Answer from the drawing. Dimensions are ordinates in mm from the lowest x, y and z of the part. Coordinates: 2 decimals unless noted, no trailing zeros. Write each loop counter-clockwise with the first axis right and the second up, starting at its lowest first coordinate (ties: lowest second). Pieces come first, ordered by that corner, then holes.
(1) The part is cut by section A-A on y = 1.8. Give the number of separate pieces and of enclosed holes in the cut face, plus the area to 3 significant figures.
(2) Straight lines are drawn through the part: line 1 (X direction, y = 0.6, z = 74.5) (1 decimal); line 2 (Z direction, x = 269, y = 0.55) (1 decimal). For each, find the intervals that lie inside material, in ascending order.
(3) Given P1, Ø1.6, axis at x = 264.5, y = 2, coming from the -Z side (3 decimals); P2, Ø1, axis at y = 2, z = 1, coming from the +X side; P3, Ø1.6, axis at x = 1.5, y = 1.5, coming from the -Z side (3 decimals), each flat-ended and moving along its own axis, determine where each tip first touches the part or whether it passes through.
(4) The part is cut by section B-B on z = 39. Determine the outline of the cut face in (x, y) (1 decimal).
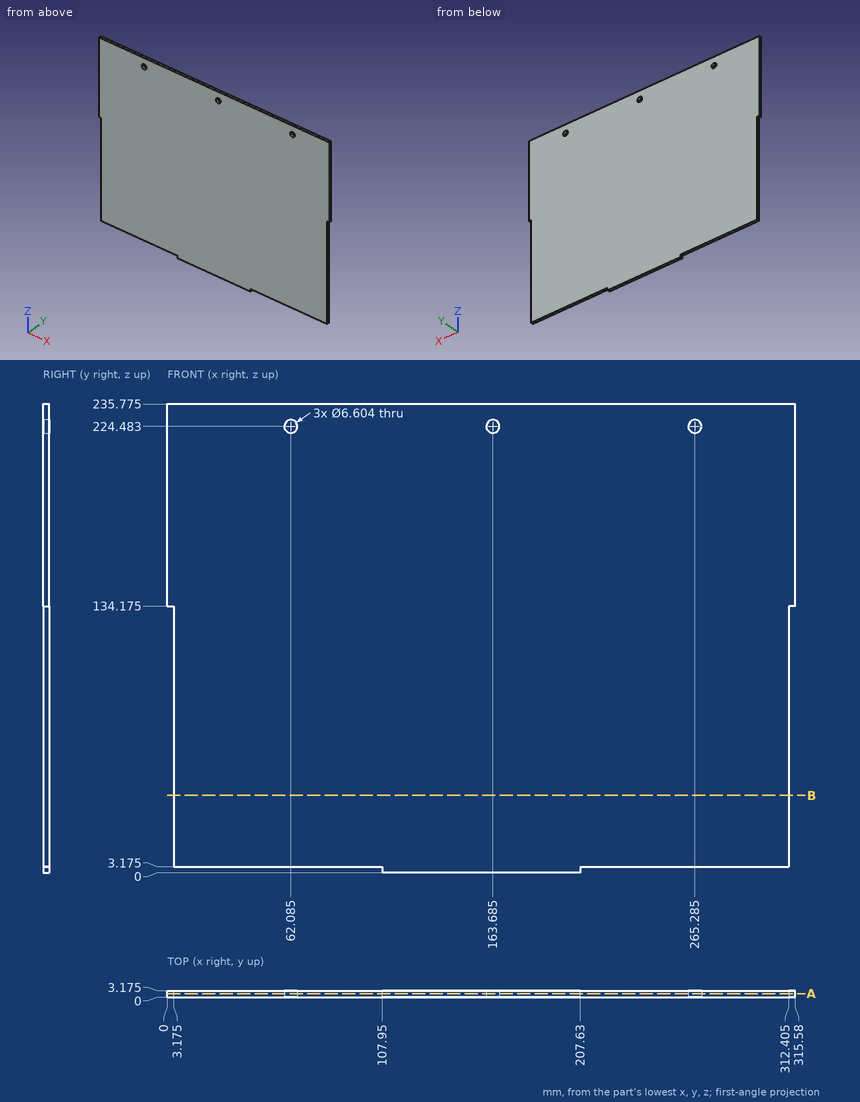
Model answer:
1. separate pieces: 1
1. enclosed holes: 3
1. area: 72,800 mm2
2. line 1: x = 3.2 to 312.4
2. line 2: z = 3.2 to 235.8
3. P1: stops at z = 3.175
3. P2: stops at x = 207.63
3. P3: stops at z = 134.175
4. outline: (3.2, 0) - (312.4, 0) - (312.4, 3.2) - (3.2, 3.2) - close
